Print and shaded views of the part. All mm, measured from the part's lowest x, y and z. A direction names the side the tool comes from. Round coordinates to 2 decimals unless told otherwise and drop trailing zeros. Write each loop counter-clockwise with the first axis right and the second up, starting at its lowest first coordinate (ties: lowest second). Pieces come first, ordered by that corner, then holes. Notation, with made-up numbers: (49, 26) - (63, 26) arc R18 cw to (63, 39) - close; hole circle Ø8 at (-26.75, 22). An arc over 180 degrees is marked (long way). Answer as a JSON object with one key per item and string values. Group by question number.
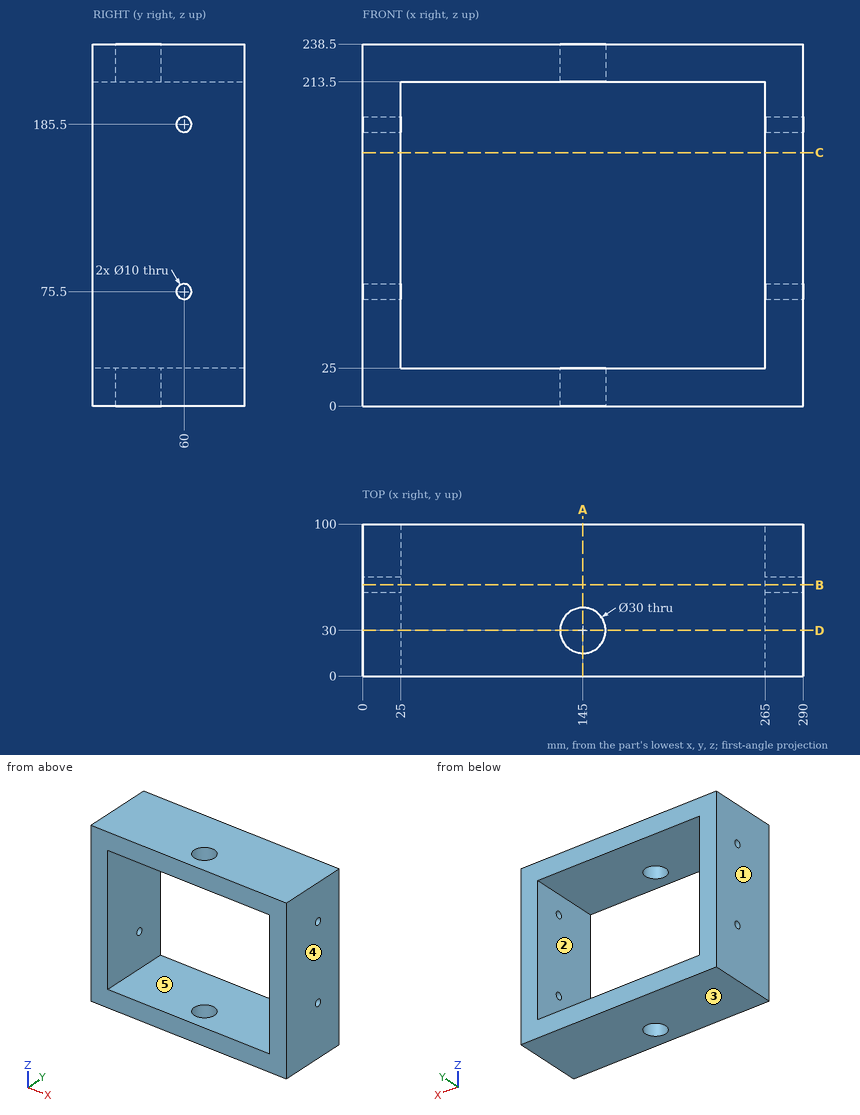
(1) Slice it at B-B (y = 60). Write the cut outline in (x, z), then the cut area to 3 significant figures.
(2) Drill centre lines: line 1 (Z direction, x = 9, y = 60); line 2 (Z direction, x = 256.5, y = 68); line 3 (X direction, y = 7, z = 34). Where is each one in solid material? Low to high. Write a range as from..to.
(3) 3-axis set-ups, long thin cutter, end or side, ignore diameter. For the marked faces 1 and 2: which of +Z, -Z, +X, -X, +Y, -Y reach the whole face in a straight line?
(4) Flat gauge pin, fed straight in: pin 1 (9 mm diameter, centred on y = 60, z = 185.5, fed in from +X). Where does the tip first touch, or does it go through?
(5) Slice it at C-C (z = 167). Write the cut outline in (x, y), then the cut area to 3 significant figures.
(6) Slice it at A-A (x = 145). Write the cut outline in (y, z).
(7) Slice it at D-D (y = 30). Write the cut outline in (x, z), then the cut area to 3 significant figures.
(8) Pull direction Z, two halves, no side cores. Call the marked faces 3, 4 and 5: pulls with the +Z half, pulls with the -Z half, needs draft (parallel to the pull), parting line crosses it, or undercut.
Answer:
{
 "1": {"outline": "(0, 0) - (290, 0) - (290, 70.5) - (265, 70.5) - (265, 25) - (25, 25) - (25, 70.5) - (0, 70.5) - close; (0, 80.5) - (25, 80.5) - (25, 180.5) - (0, 180.5) - close; (0, 190.5) - (25, 190.5) - (25, 213.5) - (265, 213.5) - (265, 190.5) - (290, 190.5) - (290, 238.5) - (0, 238.5) - close; (265, 80.5) - (290, 80.5) - (290, 180.5) - (265, 180.5) - close", "area": "22,900 mm²"},
 "2": {"line 1": "0..70.5, 80.5..180.5, 190.5..238.5", "line 2": "0..25, 213.5..238.5", "line 3": "0..25, 265..290"},
 "3": {"face 1": "+Z, -Z, -X, +Y, -Y", "face 2": "+Y, -Y"},
 "4": {"pin 1": "through"},
 "5": {"outline": "(0, 0) - (25, 0) - (25, 100) - (0, 100) - close; (265, 0) - (290, 0) - (290, 100) - (265, 100) - close", "area": "5,000 mm²"},
 "6": {"outline": "(0, 0) - (15, 0) - (15, 25) - (0, 25) - close; (0, 213.5) - (15, 213.5) - (15, 238.5) - (0, 238.5) - close; (45, 0) - (100, 0) - (100, 25) - (45, 25) - close; (45, 213.5) - (100, 213.5) - (100, 238.5) - (45, 238.5) - close"},
 "7": {"outline": "(0, 0) - (130, 0) - (130, 25) - (25, 25) - (25, 213.5) - (130, 213.5) - (130, 238.5) - (0, 238.5) - close; (160, 0) - (290, 0) - (290, 238.5) - (160, 238.5) - (160, 213.5) - (265, 213.5) - (265, 25) - (160, 25) - close", "area": "22,400 mm²"},
 "8": {"face 3": "pulls with the -Z half", "face 4": "needs draft", "face 5": "undercut"}
}
